from build123d import *

# Parameters (mm, degrees)
SKETCH1_R           = 72.5
BOSS_EXTRUDE1_DEPTH = 13
SKETCH2_R           = 30
CUT_EXTRUDE1_DEPTH  = 104.351342517
SKETCH3_R           = 7.618751991
CUT_EXTRUDE2_DEPTH  = 12.55665
CIRPATTERN1_START   = 0.443350463
CIRPATTERN1_DEPTH   = 12.556649537


# Read off the part's stored shape, not the designer's step: CirPattern1
with BuildPart() as part:
    # Sketch1 → Boss-Extrude1 (new body)
    with BuildSketch(Plane(origin=(0, 0, 0), x_dir=(1, 0, 0), z_dir=(0, 1, 0))):
        with Locations(Location((0, 0, 0), (0, 0, 90))):
            Circle(SKETCH1_R)
    extrude(amount=BOSS_EXTRUDE1_DEPTH)

    # Sketch2 → Cut-Extrude1 (cut, through all)
    with BuildSketch(Plane(origin=(0, 0, 0), x_dir=(1, 0, 0), z_dir=(0, 1, 0))):
        with Locations(Location((0, 0, 0), (0, 0, 90))):
            Circle(SKETCH2_R)
    extrude(amount=CUT_EXTRUDE1_DEPTH, mode=Mode.SUBTRACT)

    # Sketch3 → Cut-Extrude2 (cut)
    with BuildSketch(Plane(origin=(0, 13, 0), x_dir=(1, 0, 0), z_dir=(0, 1, 0))):
        with Locations((-31.234649967, 0)):
            Circle(SKETCH3_R)
    extrude(amount=-CUT_EXTRUDE2_DEPTH, mode=Mode.SUBTRACT)

    # CirPattern1 outline → CirPattern1 (cut)
    with BuildSketch(Plane(origin=(0, 0, 0), x_dir=(1, 0, 0), z_dir=(0, 1, 0)).offset(CIRPATTERN1_START)):
        with BuildLine():
            ThreePointArc((8.215061667, 28.853297243), (15, 25.980762114), (20.880157562, 21.541100719))
            ThreePointArc((20.880157562, 21.541100719), (19.426700979, 33.648033119), (8.215061667, 28.853297243))
        make_face()
        with BuildLine():
            ThreePointArc((20.880157562, -21.541100719), (15, -25.980762114), (8.215061667, -28.853297243))
            ThreePointArc((8.215061667, -28.853297243), (19.426700979, -33.648033119), (20.880157562, -21.541100719))
        make_face()
    extrude(amount=CIRPATTERN1_DEPTH, mode=Mode.SUBTRACT)


solid = part.part
Work out the finished part from the listing and answer in its coordinate system (mm). A direction names the side the tool comes from. Give positions to 0.01 mm unless a question says otherwise; leave off trailing zeros. Write each loop counter-clockwise with the first axis right and the second up, starting at its lowest first coordinate (ties: lowest second). Pieces come first, ordered by that corner, then holes. Notation, with made-up numbers: (73.5, -36) - (120.5, -36) arc R32 ccw to (120.5, 1) - close; hole circle Ø3 at (-26, 34.25). An arc over 180 degrees is marked (long way). One line per item, written item: value. Start each with the question number.
1. Find section B-B (x = 0). Write down the section's boundary in (y, z).
2. For a pull along X with two mould halves and no side action, classify faces 1 (the cylindrical face through (-21.78, 6.41, -69.15)), 2 (the flat face through (-1, 13, -31)), 3 (the cylindrical face through (19.597, 6.634, -33.547)) as +X half, -X half, draft (parallel to the pull), parting line (faces both ways), or undercut.
3. Find section D-D (z = -26). Write down the section's boundary in (x, y).
4. Given pin 1 (3 mm diameter, centred on y = 10.5, z = -30.5, fed in from -X); pin 2 (4 mm diameter, centred on x = 18, z = -26.5, fed in from +Y); pin 3 (1 mm diameter, centred on y = 4, z = -52.5, fed in from -X), each flat-ended and moving along its own axis, determine where each tip first touches the part or whether it passes through.
5. Consider probe 1 along Z at (x, y) = (-1, 7.5); probe 2 along X at (y, z) = (12, -8.5); probe 3 along Y at (x, z) = (-34, 5). Determine where each line is inside the solid, lowest interval first.
6. For faces 4 (the cylindrical face through (26.615, 6.409, -13.843)), 5 (the flat face through (17, 0.443, 29)), determine the directions among +Z, -Z, +X, -X, +Y, -Y from which every point of the face is accessible in a straight line to the end or side of a thin tool.
7. Find section A-A (z = 0). Write down the section's boundary in (x, y), then the cut area to 3 significant figures.
8. Find section C-C (y = 9.5). Write down the section's boundary in (x, z).
Geometry results:
1. outline: (0, -72.5) - (13, -72.5) - (13, -30) - (0, -30) - close; (0, 30) - (13, 30) - (13, 72.5) - (0, 72.5) - close
2. face 1: parting line
2. face 2: draft
2. face 3: undercut
3. outline: (-67.68, 0) - (-14.97, 0) - (-14.97, 13) - (-67.68, 13) - close; (14.97, 0) - (67.68, 0) - (67.68, 13) - (23.16, 13) - (23.16, 0.44) - (14.97, 0.44) - close
4. pin 1: x = -66.45
4. pin 2: y = 0.44
4. pin 3: x = -50.52
5. probe 1: -72.49 to -29.98, 29.98 to 72.49
5. probe 2: -72 to -28.77, 28.77 to 72
5. probe 3: 0 to 0.44
6. face 4: +Y, -Y
6. face 5: +Y
7. outline: (-72.5, 0) - (-30, 0) - (-30, 0.44) - (-38.85, 0.44) - (-38.85, 13) - (-72.5, 13) - close; (30, 0) - (72.5, 0) - (72.5, 13) - (30, 13) - close
7. area: 994 mm2
8. outline: circle Ø145 at (0, 0); hole (-29.1, -7.31) arc R30 ccw to (8.22, -28.85) arc R7.62 ccw (long way) to (20.88, -21.54) arc R30 ccw to (20.88, 21.54) arc R7.62 ccw (long way) to (8.22, 28.85) arc R30 ccw to (-29.1, 7.31) arc R7.62 ccw (long way) to start
